from build123d import *

# Parameters (mm, degrees)
SKETCH020_W     = 6
SKETCH020_H     = 60
PAD004_DEPTH    = 31
SKETCH021_R     = 11.2
POCKET_DEPTH    = 6.001
FILLET004_R     = 1
SKETCH027_R     = 0.75
POCKET009_DEPTH = 12


with BuildPart() as part:
    # Sketch020 → Pad004 (new body)
    with BuildSketch(Plane.XY):
        with Locations((70, 5)):
            Rectangle(SKETCH020_W, SKETCH020_H)
    extrude(amount=PAD004_DEPTH)

    # Sketch021 → Pocket (cut, through all)
    with BuildSketch(Plane.YZ.offset(73)):
        with Locations((5, 31)):
            Circle(SKETCH021_R)
    extrude(amount=-POCKET_DEPTH, mode=Mode.SUBTRACT)

    # Fillet004
    fillet004_edges = [part.edges().sort_by_distance(p)[0] for p in [
        (73, -25, 15.5),
        (67, -25, 15.5),
        (70, -25, 0),
        (70, -25, 31),
        (67, 35, 15.5),
        (73, 35, 15.5),
        (70, 35, 0),
        (70, 35, 31),
    ]]
    fillet(fillet004_edges, radius=FILLET004_R)

    # Sketch027 → Pocket009 (cut)
    with BuildSketch(Plane.XY.offset(31)):
        with Locations((70, 25.1)):
            Circle(SKETCH027_R)
        with Locations((70, -15.1)):
            Circle(SKETCH027_R)
    extrude(amount=-POCKET009_DEPTH, mode=Mode.SUBTRACT)


solid = part.part
Work out the finished part from the listing and answer in its coordinate system (mm). A direction names the side the tool comes from. Round coordinates to 2 decimals unless told otherwise and drop trailing zeros. Write each loop counter-clockwise with the first axis right and the second up, starting at its lowest first coordinate (ties: lowest second). Pieces come first, ordered by that corner, then holes. Notation, with made-up numbers: (3, 30) - (7, 30) arc R12 ccw to (7, 37) - close; hole circle Ø1 at (20.5, 44). An arc over 180 degrees is marked (long way). Answer in a Markdown table with one row per item. Add a question column.
1. A cutting plane is placed at D-D, the plane z = 26. Determine the outline of the cut face in (x, y).
2. For faces 5 (the cylindrical face through (69.25, -15.07, 25.08)), 6 (the cylindrical face through (70, 4.8, 19.8)), determine the directions among +Z, -Z, +X, -X, +Y, -Y from which every point of the face is accessible in a straight line to the end or side of a thin tool.
3. The mould has two halves that part along X. Classify faces 1 (the cylindrical face through (69.25, 25.13, 25.08)), 2 (the flat face through (67, 5, 15)), 3 (the flat face through (70, -15, 19)), 4 (the flat face through (69, -15, 31)): +X half, -X half, draft (parallel to the pull), parting line (faces both ways), or undercut.
4. A cutting plane is placed at C-C, the plane y = -15.1. Determine the outline of the cut face in (x, z), and give its area (3 significant figures).
5. Find the intervals of material crossed by line 1 along X through (y, z) = (25, 26); line 2 along Y through (x, z) = (70, 27); line 3 along Y through (x, z) = (70, 25), in increasing order. Write a range as from..to.
6. A cutting plane is placed at B-B, the plane x = 68.7. Determine the outline of the cut face in (y, z).
7. Given pin 1 (1.2 mm diameter, centred on x = 70, y = -15.1, fed in from +Z), flat-ended and moving along its own axis, determine where the tip first touches the part or whether it passes through.
8. A cutting plane is placed at A-A, the plane z = 22.5. Determine the outline of the cut face in (x, y), and give its area (3 significant figures).
Worked out:
| question | item | result |
|---|---|---|
| 1 | outline | (67, -24) arc R1 ccw to (68, -25) - (72, -25) arc R1 ccw to (73, -24) - (73, -5.02) - (67, -5.02) - close; (67, 15.02) - (73, 15.02) - (73, 34) arc R1 ccw to (72, 35) - (68, 35) arc R1 ccw to (67, 34) - close; hole circle Ø1.5 at (70, -15.1); hole circle Ø1.5 at (70, 25.1) |
| 2 | face 5 | +Z |
| 2 | face 6 | +Z, +X, -X |
| 3 | face 1 | undercut |
| 3 | face 2 | -X half |
| 3 | face 3 | undercut |
| 3 | face 4 | draft |
| 4 | outline | (67, 0) - (73, 0) - (73, 31) - (70.75, 31) - (70.75, 19) - (69.25, 19) - (69.25, 31) - (67, 31) - close |
| 4 | area | 168 mm^2 |
| 5 | line 1 | 67..69.26, 70.74..73 |
| 5 | line 2 | -25..-15.85, -14.35..-5.46, 15.46..24.35, 25.85..35 |
| 5 | line 3 | -25..-15.85, -14.35..-4.46, 14.46..24.35, 25.85..35 |
| 6 | outline | (-25, 1) arc R1 ccw to (-24, 0) - (34, 0) arc R1 ccw to (35, 1) - (35, 30) arc R1 ccw to (34, 31) - (16.2, 31) arc R11.2 cw to (-6.2, 31) - (-24, 31) arc R1 ccw to (-25, 30) - close |
| 7 | pin 1 | z = 19 |
| 8 | outline | (67, -24) arc R1 ccw to (68, -25) - (72, -25) arc R1 ccw to (73, -24) - (73, -2.29) - (67, -2.29) - close; (67, 12.29) - (73, 12.29) - (73, 34) arc R1 ccw to (72, 35) - (68, 35) arc R1 ccw to (67, 34) - close; hole circle Ø1.5 at (70, -15.1); hole circle Ø1.5 at (70, 25.1) |
| 8 | area | 268 mm^2 |
